Input: dimensioned drawing with shaded views. Units: mm. Origin: part minimum x, y, z. Give positions to 0.01 mm unless a question says otherwise; leave off trailing zeros. Write each loop counter-clockwise with the first axis right and the second up, starting at its lowest first coordinate (ties: lowest second). Pieces come first, ordered by that corner, then holes. Notation, with made-up numbers: M 46,-38.75 L 104,-38.75 A31 ccw 104,-13.75 Z; hole C 3.25,54 d8. An arc over 180 degrees is marked long. Answer as a JSON object with one key per item and string values.
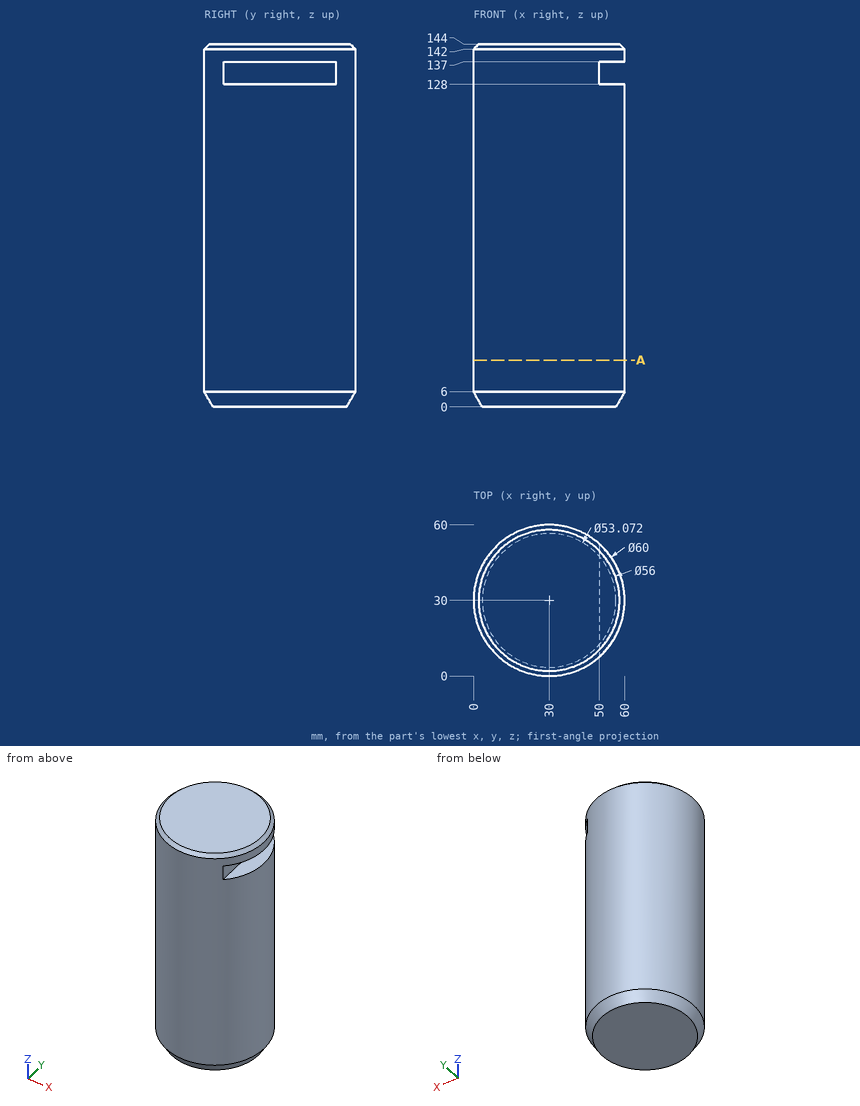
1) Line query: line 1 (Z direction, x = 52, y = 28.5); line 2 (Y direction, x = 44, z = 84); line 3 (Y direction, x = 5.5, z = 7). Output: solid intervals per line, ascending. Write a range as from..to.
Geometry check:
{"line 1": "z = 0..128, 137..144", "line 2": "y = 3.47..56.53", "line 3": "y = 12.69..47.31"}
2) Contact query for flat-ended pins moving along their axis: P1, Ø4.5, axis at y = 39, z = 131, coming from the +X side; P2, Ø1, axis at y = 19, z = 94.5, coming from the -X side; P3, Ø4, axis at x = 54, z = 100.5, coming from the -Y side. Output: stop coordinate, or through.
Geometry check:
{"P1": "stops at x = 50", "P2": "stops at x = 1.9", "P3": "stops at y = 9.6"}
3) Cut plane A-A on z = 18.5. Return loops of the section in (x, y).
Geometry check:
{"outline": "C 30,30 d60"}
